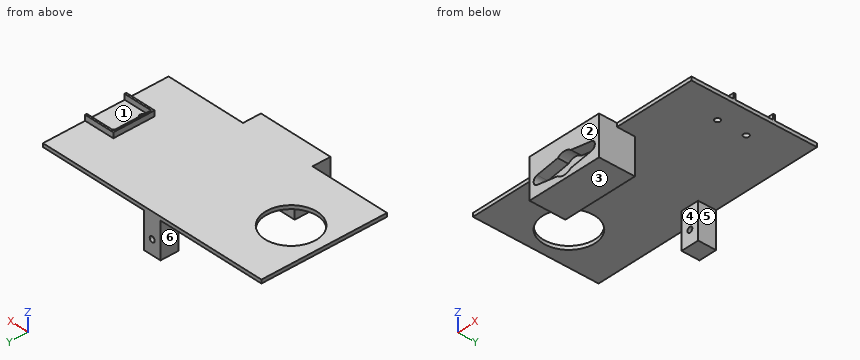
from build123d import *

# Parameters (mm, degrees)
BOSS_EXTRUDE1_DEPTH = 2
SKETCH2_R           = 14.5
CUT_EXTRUDE1_DEPTH  = 2
BOSS_EXTRUDE2_DEPTH = 3
CUT_EXTRUDE2_REACH  = 81.937
SKETCH5_R           = 1.5
SKETCH6_W           = 10
SKETCH6_H           = 10
BOSS_EXTRUDE3_DEPTH = 20
SKETCH10_W          = 42
SKETCH10_H          = 20
BOSS_EXTRUDE5_DEPTH = 20
CUT_EXTRUDE3_DEPTH  = 6
CUT_EXTRUDE4_REACH  = 107.622
SKETCH12_R          = 1.5


with BuildPart() as part:
    # Sketch1 → Boss-Extrude1 (new body)
    with BuildSketch(Plane.XY):
        Polygon((21, -35), (66, -35), (66, 35), (-66, 35), (-66, -35), (-21, -35), (-21, -45), (21, -45), align=None)
    extrude(amount=BOSS_EXTRUDE1_DEPTH)

    # Sketch2 → Cut-Extrude1 (cut)
    with BuildSketch(Plane.XY.offset(2)):
        with Locations((-46, 0)):
            Circle(SKETCH2_R)
    extrude(amount=-CUT_EXTRUDE1_DEPTH, mode=Mode.SUBTRACT)

    # Sketch3 → Boss-Extrude2 (add)
    with BuildSketch(Plane.XY.offset(2)):
        Polygon((50, -10.5), (50, 10.5), (66, 10.5), (66, 11.5), (49, 11.5), (49, -11.5), (66, -11.5), (66, -10.5), align=None)
    extrude(amount=BOSS_EXTRUDE2_DEPTH)

    # Sketch5 → Cut-Extrude2 (cut, up to next)
    with BuildSketch(Plane.XY.offset(2), mode=Mode.PRIVATE) as cut_extrude2_sk1:
        with Locations((52.5, 8)):
            Circle(SKETCH5_R)
    cut_extrude2_tool1 = extrude(cut_extrude2_sk1.sketch, amount=-CUT_EXTRUDE2_REACH, mode=Mode.PRIVATE) & part.part
    # Sketch5 → Cut-Extrude2 (cut, up to next)
    with BuildSketch(Plane.XY.offset(2), mode=Mode.PRIVATE) as cut_extrude2_sk2:
        with Locations((52.5, -8)):
            Circle(SKETCH5_R)
    cut_extrude2_tool2 = extrude(cut_extrude2_sk2.sketch, amount=-CUT_EXTRUDE2_REACH, mode=Mode.PRIVATE) & part.part
    add(cut_extrude2_tool1.solids().sort_by_distance((52.5, 8, 2))[0], mode=Mode.SUBTRACT)
    add(cut_extrude2_tool2.solids().sort_by_distance((52.5, -8, 2))[0], mode=Mode.SUBTRACT)

    # Sketch6 → Boss-Extrude3 (add)
    with BuildSketch(Plane(origin=(0, 0, 0), x_dir=(-1, 0, 0), z_dir=(0, 0, -1))):
        with Locations((0, 30)):
            Rectangle(SKETCH6_W, SKETCH6_H)
    extrude(amount=BOSS_EXTRUDE3_DEPTH)

    # Sketch10 → Boss-Extrude5 (add)
    with BuildSketch(Plane(origin=(0, 0, 0), x_dir=(-1, 0, 0), z_dir=(0, 0, -1))):
        with Locations((0, -35)):
            Rectangle(SKETCH10_W, SKETCH10_H)
    extrude(amount=BOSS_EXTRUDE5_DEPTH)

    # Sketch11 → Cut-Extrude3 (cut)
    with BuildSketch(Plane.XZ.offset(45)):
        with BuildLine():
            Line((-3.932248681, -7.468176933), (-16.408317349, -9.533589408))
            ThreePointArc((-16.408317349, -9.533589408), (-18.5, -12.000023193), (-16.408309881, -14.466450643))
            Line((-16.408309881, -14.466450643), (-3.932248681, -16.531823067))
            ThreePointArc((-3.932248681, -16.531823067), (0, -18), (3.932248681, -16.531823067))
            Line((3.932248681, -16.531823067), (16.408313615, -14.466430618))
            ThreePointArc((16.408313615, -14.466430618), (18.5, -12), (16.408313615, -9.533569382))
            Line((16.408313615, -9.533569382), (3.932248681, -7.468176933))
            ThreePointArc((3.932248681, -7.468176933), (0, -6), (-3.932248681, -7.468176933))
        make_face()
    extrude(amount=-CUT_EXTRUDE3_DEPTH, mode=Mode.SUBTRACT)

    # Sketch12 → Cut-Extrude4 (cut, up to next)
    with BuildSketch(Plane(origin=(0, 35, 0), x_dir=(1, 0, 0), z_dir=(0, 1, 0)), mode=Mode.PRIVATE) as cut_extrude4_sk1:
        with Locations(Location((0, 12, 0), (0, 0, 270))):
            Circle(SKETCH12_R)
    cut_extrude4_tool1 = extrude(cut_extrude4_sk1.sketch, amount=-CUT_EXTRUDE4_REACH, mode=Mode.PRIVATE) & part.part
    add(cut_extrude4_tool1.solids().sort_by_distance((0, 35, -12))[0], mode=Mode.SUBTRACT)


solid = part.part
The model under review builds one solid part; all positions refer to its coordinate system, in mm. Face numbers are marked on the shaded views. A direction names the side the tool comes from. Give positions to 0.01 mm unless a question says otherwise; leave off trailing zeros. Loops run counter-clockwise (first coordinate to the right, second up) from the corner with the lowest first, then second, coordinate; pieces in that order, holes last. Notation, with made-up numbers: (89.5, 12.25) -> (93.5, 12.25) arc R19 cw to (93.5, 21.25) -> close; hole circle Ø3 at (82.25, 11). An arc over 180 degrees is marked (long way). Put each result on its own line as item: value. Start each with the question number.
1. We need section C-C on y = 8. State the section outline as (x, z) points.
2. We need section A-A on x = 0. State the section outline as (y, z) points, then the cut area to 3 significant figures.
3. Mouldability with a two-part tool opening along Y and no side actions: class the marked faces 1, 2 and 3 as released by +Y, released by -Y, zero draft, split by the parting line, or undercut.
4. We need section D-D on x = -46. State the section outline as (y, z) points, then the cut area to 3 significant figures.
5. Wall thickness on probe 1 along Y at (x, z) = (52.5, 1.1); probe 2 along Y at (x, z) = (-46, 1.45); probe 3 along Y at (x, z) = (53, 3.75): over which ranges is each line inside the solid? List them lowest first.
6. For the marked faces 4, 5 and 6, list the 3-axis set-ups (+Z, -Z, +X, -X, +Y, -Y) from which the entire face can be reached by the end or side of a thin tool; tool diameter is ignored.
7. Clearance check with flat-ended pins moving along their axes: P1, Ø21, axis at x = 31.5, y = 11, coming from the -Z side; P2, Ø4, axis at x = 10, z = -4, coming from the +Y side; P3, Ø0.9, axis at y = 4.5, z = 3.5, coming from the -X side; P4, Ø10, axis at y = 0.5, z = -7, coming from the -X side. State where each tip first meets the part, or that it passes through.
8. We need section B-B on z = -3.5. State the section outline as (x, y) points.
Determined:
1. outline: (-66, 0) -> (-58.09, 0) -> (-58.09, 2) -> (-66, 2) -> close; (-33.91, 0) -> (51, 0) -> (51, 2) -> (50, 2) -> (50, 5) -> (49, 5) -> (49, 2) -> (-33.91, 2) -> close; (54, 0) -> (66, 0) -> (66, 2) -> (54, 2) -> close
2. outline: (-45, -20) -> (-25, -20) -> (-25, 0) -> (25, 0) -> (25, -10.5) -> (35, -10.5) -> (35, 2) -> (-45, 2) -> (-45, -6) -> (-39, -6) -> (-39, -18) -> (-45, -18) -> close; (25, -20) -> (35, -20) -> (35, -13.5) -> (25, -13.5) -> close
2. area: 658 mm^2
3. face 1: undercut
3. face 2: released by -Y
3. face 3: zero draft
4. outline: (-35, 0) -> (-14.5, 0) -> (-14.5, 2) -> (-35, 2) -> close; (14.5, 0) -> (35, 0) -> (35, 2) -> (14.5, 2) -> close
4. area: 82.0 mm^2
5. probe 1: -35 to -9.5, -6.5 to 6.5, 9.5 to 35
5. probe 2: -35 to -14.5, 14.5 to 35
5. probe 3: -11.5 to -10.5, 10.5 to 11.5
6. face 4: -Z, +X, -X
6. face 5: -Z, +X, +Y
6. face 6: -Z, -X, +Y
7. P1: z = 0
7. P2: y = -25
7. P3: x = 49
7. P4: through
8. outline: (-21, -45) -> (21, -45) -> (21, -25) -> (-21, -25) -> close; (-5, 25) -> (5, 25) -> (5, 35) -> (-5, 35) -> close
